```python
from build123d import *

# Parameters (mm, degrees)
CORTAR_EXTRUIR1_DEPTH = 3.9
REDONDEO1_R           = 0.2


with BuildPart() as part:
    # Croquis1 → Revolución1 (revolve)
    with BuildSketch(Plane.XY):
        Polygon((0, 37.735435589), (0, -28.264564411), (-2, -28.264564411), (-2.925, -27.764564411), (-2.925, 31.835435589), (-4.875, 31.835435589), (-4.875, 37.735435589), align=None)
    revolve(axis=Axis((0, 37.735435589, 0), (0, -1, 0)))

    # Croquis2 → Cortar-Extruir1 (cut)
    with BuildSketch(Plane(origin=(0, 37.735435589, 0), x_dir=(1, 0, 0), z_dir=(0, 1, 0))):
        Polygon((2.75, 0), (1.375, 2.38156986), (-1.375, 2.38156986), (-2.75, 0), (-1.375, -2.38156986), (1.375, -2.38156986), align=None)
    extrude(amount=-CORTAR_EXTRUIR1_DEPTH, mode=Mode.SUBTRACT)

    # Redondeo1
    redondeo1_edges = [part.edges().sort_by_distance(p)[0] for p in [
        (4.875, 37.735435589, 0),
    ]]
    fillet(redondeo1_edges, radius=REDONDEO1_R)


solid = part.part
```
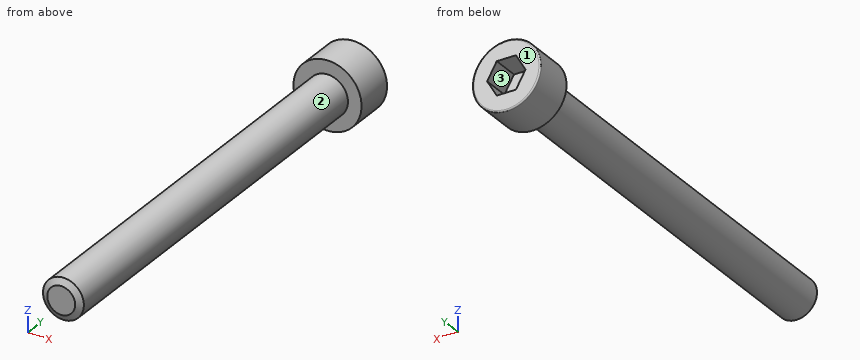
Work out the finished part from the listing and answer in its coordinate system (mm). Face numbers are marked on the shaded views. Give positions to 0.01 mm unless a question says otherwise; leave off trailing zeros. Order: outer loops, then holes, each group sorted by start corner. A loop starts at its lowest first (then second) coordinate and runs counter-clockwise, first axis right, second up. Notation, with made-up numbers: M 12.5,12 L 50.5,12 A25 cw 50.5,44 Z; hole C 24.25,85.25 d3. An arc over 180 degrees is marked long. Return JSON: item names as keys, results as strings.
1) For a pull along X with two mould halves and no side action, classify the marked faces 1, 2 and 3 as +X half, -X half, draft (parallel to the pull), parting line (faces both ways), or undercut.
Resolved:
{"face 1": "draft", "face 2": "parting line", "face 3": "undercut"}
2) Section A-A, the plane x = 0 is taken. Write down the section's boundary in (y, z) (3 decimals), plus the area to 3 significant figures.
Resolved:
{"outline": "M -28.265,-2 L -27.765,-2.925 L 31.835,-2.925 L 31.835,-4.875 L 37.535,-4.875 A0.2 ccw 37.735,-4.675 L 37.735,-2.382 L 33.835,-2.382 L 33.835,2.382 L 37.735,2.382 L 37.735,4.675 A0.2 ccw 37.535,4.875 L 31.835,4.875 L 31.835,2.925 L -27.765,2.925 L -28.265,2 Z", "area": "390 mm^2"}
3) Section B-B, the plane y = -16 is taken. Write down the section's boundary in (x, z) (3 decimals).
Resolved:
{"outline": "C 0,0 d5.85"}
4) Each of these flat-tipped pins is pushed along its axis until it touches: pin 1 (1 mm diameter, centred on x = 1.5, y = 26.5, fed in from -Z); pin 2 (2.5 mm diameter, centred on x = 0.5, z = 0, fed in from +Y); pin 3 (3 mm diameter, centred on y = 13, z = 0.5, fed in from +X) (3 decimals). Where does it stop, or does it pass through?
Resolved:
{"pin 1": "z = -2.75", "pin 2": "y = 33.84", "pin 3": "x = 2.925"}
5) Straight lines are drawn through the part: line 1 along Y through (x, z) = (-0.25, -1); line 2 along X through (y, z) = (22, 0) (3 decimals). For each, find the intervals that lie inside material, in ascending order. Write a range as [from, to].
Resolved:
{"line 1": "[-28.26, 33.84]", "line 2": "[-2.925, 2.925]"}
